The listing builds one solid part. Answer for the finished solid, in the listing's coordinates (mm). Round coordinates to 2 decimals unless told otherwise and drop trailing zeros. Order: outer loops, then holes, each group sorted by start corner. A loop starts at its lowest first (then second) coordinate and runs counter-clockwise, first axis right, second up. Notation, with made-up numbers: (15, -3) - (44, -3) arc R27 cw to (44, 32) - close; hole circle Ø5 at (0, 16.25). An arc over 180 degrees is marked (long way). One line per item, written item: value. Start each with the question number.
1. Section A-A, the plane y = -16.5 is taken. Give the vertices of the cut face in (x, z) (3 decimals).
2. Section B-B, the plane x = 0 is taken. Count the separate pieces of the cut face and the enclosed holes in it, then the cut area to 3 significant figures.
3. Section D-D, the plane y = 61.5 is taken. Give the vertices of the cut face in (x, z) (3 decimals).
4. Straight lines are drawn through the part: line 1 (X direction, y = -13, z = 2.75) (3 decimals); line 2 (X direction, y = 26.5, z = 0.7) (3 decimals); line 3 (X direction, y = 91, z = 1.95) (3 decimals). For each, find the intervals that lie inside material, in ascending order.
5. A flat-ended cylindrical pin translates along its axis: P1, Ø11.5, axis at x = -11.5, y = -46.37, coming from the +Z side (3 decimals). Find the tip coordinate at first contact, or state that the pin passes through.
from build123d import *

# Parameters (mm, degrees)
SKETCH1_W                                       = 56.55
SKETCH1_H                                       = 197.425
BOSS_EXTRUDE1_DEPTH                             = 3.175
SKETCH4_R                                       = 5
CUT_EXTRUDE2_DEPTH                              = 103.731270343
LPATTERN3_COUNT                                 = 13
LPATTERN3_PITCH                                 = 11
SKETCH5_W                                       = 3.175
SKETCH5_H                                       = 197.425
BOSS_EXTRUDE2_DEPTH                             = 19.525
SKETCH14_W                                      = 76.075
SKETCH14_H                                      = 3.175
BOSS_EXTRUDE3_DEPTH                             = 3.175
M4_CLEARANCE_HOLE1_D                            = 4.5
CSK_FOR_M3_FLAT_HEAD_MACHINE_SCREW4_D           = 3.4
CSK_FOR_M3_FLAT_HEAD_MACHINE_SCREW4_CSINK_D     = 6.3
CSK_FOR_M3_FLAT_HEAD_MACHINE_SCREW4_CSINK_ANGLE = 90


with BuildPart() as part:
    # Sketch1 → Boss-Extrude1 (new body)
    with BuildSketch(Plane.XY):
        Rectangle(SKETCH1_W, SKETCH1_H)
    extrude(amount=BOSS_EXTRUDE1_DEPTH)

    # Sketch4 → Cut-Extrude2 (cut, through all)
    with BuildSketch(Plane.XY.offset(3.175)):
        with Locations((0, -57.369162839)):
            Circle(SKETCH4_R)
        with Locations((11.5, -57.369162839)):
            Circle(SKETCH4_R)
        with Locations((-11.5, -57.369162839)):
            Circle(SKETCH4_R)
    cut_extrude2 = extrude(amount=-CUT_EXTRUDE2_DEPTH, mode=Mode.SUBTRACT)

    # LPattern3: Cut-Extrude2 ×13
    with Locations(*[(0, i * LPATTERN3_PITCH, 0) for i in range(1, LPATTERN3_COUNT)]):
        add(cut_extrude2, mode=Mode.SUBTRACT)

    # Sketch5 → Boss-Extrude2 (add)
    with BuildSketch(Plane.ZY.offset(28.275)):
        with Locations((1.5875, 0)):
            Rectangle(SKETCH5_W, SKETCH5_H)
    extrude(amount=BOSS_EXTRUDE2_DEPTH)

    # Sketch14 → Boss-Extrude3 (add)
    with BuildSketch(Plane(origin=(0, 98.7125, 0), x_dir=(1, 0, 0), z_dir=(0, 1, 0))):
        with Locations((-9.7625, -1.5875)):
            Rectangle(SKETCH14_W, SKETCH14_H)
    extrude(amount=BOSS_EXTRUDE3_DEPTH)

    # M4 Clearance Hole1 (through all)
    with Locations(Plane.XY.offset(3.175)):
        with Locations((0, 92.3625001), (0, -78.8874999)):
            Hole(M4_CLEARANCE_HOLE1_D / 2)

    # CSK for M3 Flat Head Machine Screw4 (through all)
    with Locations(Plane.XY.offset(3.175)):
        with Locations((17.4625, -78.8874999), (-17.4625, 92.3625001)):
            CounterSinkHole(CSK_FOR_M3_FLAT_HEAD_MACHINE_SCREW4_D / 2, CSK_FOR_M3_FLAT_HEAD_MACHINE_SCREW4_CSINK_D / 2, counter_sink_angle=CSK_FOR_M3_FLAT_HEAD_MACHINE_SCREW4_CSINK_ANGLE)


solid = part.part
Answer list:
1. outline: (-47.8, 0) - (-15.398, 0) - (-15.398, 3.175) - (-47.8, 3.175) - close; (-7.602, 0) - (-3.898, 0) - (-3.898, 3.175) - (-7.602, 3.175) - close; (3.898, 0) - (7.602, 0) - (7.602, 3.175) - (3.898, 3.175) - close; (15.398, 0) - (28.275, 0) - (28.275, 3.175) - (15.398, 3.175) - close
2. separate pieces: 16
2. enclosed holes: 0
2. area: 196 mm²
3. outline: (-47.8, 0) - (-16.023, 0) - (-16.023, 3.175) - (-47.8, 3.175) - close; (-6.977, 0) - (-4.523, 0) - (-4.523, 3.175) - (-6.977, 3.175) - close; (4.523, 0) - (6.977, 0) - (6.977, 3.175) - (4.523, 3.175) - close; (16.023, 0) - (28.275, 0) - (28.275, 3.175) - (16.023, 3.175) - close
4. line 1: x = -47.8 to -16.486, -6.514 to -4.986, 4.986 to 6.514, 16.486 to 28.275
4. line 2: x = -47.8 to -14.317, -8.683 to -2.817, 2.817 to 8.683, 14.317 to 28.275
4. line 3: x = -47.8 to -18.822, -16.103 to -1.791, 1.791 to 28.275
5. P1: stops at z = 3.175
